from build123d import *

# Parameters (mm, degrees)
CYLINDER1964_R               = 1.5
CYLINDER1964_DEPTH           = 50
CYLINDER1964_PLACEMENT_ANGLE = 45
CYLINDER1965_R               = 1.5
CYLINDER1965_DEPTH           = 50
CYLINDER1965_PLACEMENT_ANGLE = 45
CYLINDER1963_R               = 1.5
CYLINDER1963_DEPTH           = 50
CYLINDER1963_PLACEMENT_ANGLE = 45
CYLINDER1962_R               = 1.5
CYLINDER1962_DEPTH           = 50
CYLINDER1962_PLACEMENT_ANGLE = 45
CYLINDER1967_R               = 1.5
CYLINDER1967_DEPTH           = 50
CYLINDER1967_PLACEMENT_ANGLE = 45
CYLINDER1966_R               = 1.5
CYLINDER1966_DEPTH           = 50
CYLINDER1966_PLACEMENT_ANGLE = 45
CYLINDER1954_R               = 3
CYLINDER1954_DEPTH           = 3
CYLINDER1954_PLACEMENT_ANGLE = 45
CYLINDER1953_R               = 3
CYLINDER1953_DEPTH           = 3
CYLINDER1953_PLACEMENT_ANGLE = 45
CYLINDER1955_R               = 3
CYLINDER1955_DEPTH           = 3
CYLINDER1955_PLACEMENT_ANGLE = 45
CYLINDER1952_R               = 3
CYLINDER1952_DEPTH           = 3
CYLINDER1952_PLACEMENT_ANGLE = 45
CYLINDER1950_R               = 3
CYLINDER1950_DEPTH           = 3
CYLINDER1950_PLACEMENT_ANGLE = 45
CYLINDER1951_R               = 3
CYLINDER1951_DEPTH           = 3
CYLINDER1951_PLACEMENT_ANGLE = 45
CYLINDER1936_R               = 8
CYLINDER1936_DEPTH           = 6
BOX803_W                     = 148
BOX803_H                     = 40
BOX803_DEPTH                 = 40
CYLINDER1935_R               = 34
CYLINDER1935_DEPTH           = 6
CHAMFER065_SIZE              = 2


with BuildPart() as obj1:
    # Cylinder1964 → Cylinder1964 (new body)
    with BuildSketch(Plane.XY):
        Circle(CYLINDER1964_R)
    extrude(amount=CYLINDER1964_DEPTH)


with BuildPart() as obj1_1:
    # Cylinder1964 placement: moved
    add(obj1.part.moved(Location((20, 137, 0))).rotate(Axis((20, 137, 0), (0, 0, 1)), CYLINDER1964_PLACEMENT_ANGLE))


with BuildPart() as compound991:
    # Cylinder1965 → Cylinder1965 (new body)
    with BuildSketch(Plane.XY):
        Circle(CYLINDER1965_R)
    extrude(amount=CYLINDER1965_DEPTH)


with BuildPart() as compound991_1:
    # Cylinder1965 placement: moved
    add(compound991.part.moved(Location((-20, 137, 0))).rotate(Axis((-20, 137, 0), (0, 0, 1)), CYLINDER1965_PLACEMENT_ANGLE))

    # Compound991: union obj1
    add(obj1_1.part)


with BuildPart() as obj2:
    # Cylinder1963 → Cylinder1963 (new body)
    with BuildSketch(Plane.XY):
        Circle(CYLINDER1963_R)
    extrude(amount=CYLINDER1963_DEPTH)


with BuildPart() as obj2_1:
    # Cylinder1963 placement: moved
    add(obj2.part.moved(Location((31, 131, 0))).rotate(Axis((31, 131, 0), (0, 0, 1)), CYLINDER1963_PLACEMENT_ANGLE))


with BuildPart() as compound992:
    # Cylinder1962 → Cylinder1962 (new body)
    with BuildSketch(Plane.XY):
        Circle(CYLINDER1962_R)
    extrude(amount=CYLINDER1962_DEPTH)


with BuildPart() as compound992_1:
    # Cylinder1962 placement: moved
    add(compound992.part.moved(Location((-31, 131, 0))).rotate(Axis((-31, 131, 0), (0, 0, 1)), CYLINDER1962_PLACEMENT_ANGLE))

    # Compound992: union obj2
    add(obj2_1.part)


with BuildPart() as obj3:
    # Cylinder1967 → Cylinder1967 (new body)
    with BuildSketch(Plane.XY):
        Circle(CYLINDER1967_R)
    extrude(amount=CYLINDER1967_DEPTH)


with BuildPart() as obj3_1:
    # Cylinder1967 placement: moved
    add(obj3.part.moved(Location((31, 101, 0))).rotate(Axis((31, 101, 0), (0, 0, 1)), CYLINDER1967_PLACEMENT_ANGLE))


with BuildPart() as compound994:
    # Cylinder1966 → Cylinder1966 (new body)
    with BuildSketch(Plane.XY):
        Circle(CYLINDER1966_R)
    extrude(amount=CYLINDER1966_DEPTH)


with BuildPart() as compound994_1:
    # Cylinder1966 placement: moved
    add(compound994.part.moved(Location((-31, 101, 0))).rotate(Axis((-31, 101, 0), (0, 0, 1)), CYLINDER1966_PLACEMENT_ANGLE))

    # Compound993: union obj3
    add(obj3_1.part)

    # Compound994: union Compound991, Compound992
    add(compound991_1.part)
    add(compound992_1.part)


with BuildPart() as obj4:
    # Cylinder1954 → Cylinder1954 (new body)
    with BuildSketch(Plane.XY):
        Circle(CYLINDER1954_R)
    extrude(amount=CYLINDER1954_DEPTH)


with BuildPart() as obj4_1:
    # Cylinder1954 placement: moved
    add(obj4.part.moved(Location((31, 131, 0))).rotate(Axis((31, 131, 0), (0, 0, 1)), CYLINDER1954_PLACEMENT_ANGLE))


with BuildPart() as compound982:
    # Cylinder1953 → Cylinder1953 (new body)
    with BuildSketch(Plane.XY):
        Circle(CYLINDER1953_R)
    extrude(amount=CYLINDER1953_DEPTH)


with BuildPart() as compound982_1:
    # Cylinder1953 placement: moved
    add(compound982.part.moved(Location((-31, 131, 0))).rotate(Axis((-31, 131, 0), (0, 0, 1)), CYLINDER1953_PLACEMENT_ANGLE))

    # Compound982: union obj4
    add(obj4_1.part)


with BuildPart() as compound982_2:
    # Compound982 placement: moved
    add(compound982_1.part.moved(Location((0, 0, 25))))


with BuildPart() as obj5:
    # Cylinder1955 → Cylinder1955 (new body)
    with BuildSketch(Plane.XY):
        Circle(CYLINDER1955_R)
    extrude(amount=CYLINDER1955_DEPTH)


with BuildPart() as obj5_1:
    # Cylinder1955 placement: moved
    add(obj5.part.moved(Location((31, 101, 0))).rotate(Axis((31, 101, 0), (0, 0, 1)), CYLINDER1955_PLACEMENT_ANGLE))


with BuildPart() as compound984:
    # Cylinder1952 → Cylinder1952 (new body)
    with BuildSketch(Plane.XY):
        Circle(CYLINDER1952_R)
    extrude(amount=CYLINDER1952_DEPTH)


with BuildPart() as compound984_1:
    # Cylinder1952 placement: moved
    add(compound984.part.moved(Location((-31, 101, 0))).rotate(Axis((-31, 101, 0), (0, 0, 1)), CYLINDER1952_PLACEMENT_ANGLE))

    # Compound984: union obj5
    add(obj5_1.part)


with BuildPart() as compound984_2:
    # Compound984 placement: moved
    add(compound984_1.part.moved(Location((0, 0, 21))))


with BuildPart() as obj6:
    # Cylinder1950 → Cylinder1950 (new body)
    with BuildSketch(Plane.XY):
        Circle(CYLINDER1950_R)
    extrude(amount=CYLINDER1950_DEPTH)


with BuildPart() as obj6_1:
    # Cylinder1950 placement: moved
    add(obj6.part.moved(Location((20, 137, 0))).rotate(Axis((20, 137, 0), (0, 0, 1)), CYLINDER1950_PLACEMENT_ANGLE))


with BuildPart() as compound985:
    # Cylinder1951 → Cylinder1951 (new body)
    with BuildSketch(Plane.XY):
        Circle(CYLINDER1951_R)
    extrude(amount=CYLINDER1951_DEPTH)


with BuildPart() as compound985_1:
    # Cylinder1951 placement: moved
    add(compound985.part.moved(Location((-20, 137, 0))).rotate(Axis((-20, 137, 0), (0, 0, 1)), CYLINDER1951_PLACEMENT_ANGLE))

    # Compound983: union obj6
    add(obj6_1.part)


with BuildPart() as compound985_2:
    # Compound983 placement: moved
    add(compound985_1.part.moved(Location((0, 0, 25))))

    # Compound985: union Compound982, Compound984
    add(compound982_2.part)
    add(compound984_2.part)


with BuildPart() as obj7:
    # Cylinder1936 → Cylinder1936 (new body)
    with BuildSketch(Plane(origin=(0, 83, 25), x_dir=(1, 0, 0), z_dir=(0, 0, 1))):
        Circle(CYLINDER1936_R)
    extrude(amount=CYLINDER1936_DEPTH)


with BuildPart() as krychle803:
    # Box803 → Box803 (new body)
    with BuildSketch(Plane(origin=(-74, 46, 16), x_dir=(1, 0, 0), z_dir=(0, 0, 1))):
        with Locations((74, 20)):
            Rectangle(BOX803_W, BOX803_H)
    extrude(amount=BOX803_DEPTH)


with BuildPart() as cut622:
    # Cylinder1935 → Cylinder1935 (new body)
    with BuildSketch(Plane(origin=(0, 101, 21), x_dir=(1, 0, 0), z_dir=(0, 0, 1))):
        Circle(CYLINDER1935_R)
    extrude(amount=CYLINDER1935_DEPTH)

    # Cut615: cut Krychle803
    add(krychle803.part, mode=Mode.SUBTRACT)

    # Cut616: cut obj7
    add(obj7.part, mode=Mode.SUBTRACT)

    # Chamfer065
    chamfer065_edges = [cut622.edges().sort_by_distance(p)[0] for p in [
        (-7.700067, 134.116597, 21),
    ]]
    chamfer(chamfer065_edges, length=CHAMFER065_SIZE)

    # Cut619: cut Compound985
    add(compound985_2.part, mode=Mode.SUBTRACT)

    # Cut622: cut Compound994
    add(compound994_1.part, mode=Mode.SUBTRACT)


solid = cut622.part
Verification items for the finished model (mm, model axes). A direction names the side the tool comes from. Round coordinates to 2 decimals unless told otherwise and drop trailing zeros. Write each loop counter-clockwise with the first axis right and the second up, starting at its lowest first coordinate (ties: lowest second). Pieces come first, ordered by that corner, then holes.
(1) Section check A-A (x = 0). Enter the section's corners in (y, z).
Returned:
outline: (86, 21) - (133, 21) - (135, 23) - (135, 27) - (91, 27) - (91, 25) - (86, 25) - close
(2) Access from +Z, -Z, +X, -X, +Y, -Y to the whole of each face (thin tool, end or side, straight path). Record for faces 1 (the flat face through (0, 86, 24)), 2 (the flat face through (0, 88, 25)), 3 (the flat face through (33, 101, 24)).
Returned:
face 1: +Z, -Z, +X, -X, -Y
face 2: +Z, -Y
face 3: -Z
(3) Material ranges on line 1 (X direction, y = 101, z = 24.65); line 2 (X direction, y = 98.5, z = 23.5); line 3 (Y direction, x = 1, z = 24.5), recorded low to high.
Returned:
line 1: x = -34 to -32.5, -29.5 to 29.5, 32.5 to 34
line 2: x = -33.91 to -32.66, -29.34 to 29.34, 32.66 to 33.91
line 3: y = 86 to 134.99
(4) Mould release check, pull along Y, two halves, no side actions. Record for faces 4 (the conical face through (31.767, 92.978, 21.764)), 5 (the cylindrical face through (0.965, 134.986, 24.972)), 6 (the cylindrical face through (-31.196, 99.513, 25.479)): pulls with the +Y half, pulls with the -Y half, needs draft (parallel to the pull), parting line crosses it, or undercut.
Returned:
face 4: pulls with the -Y half
face 5: parting line crosses it
face 6: undercut
(5) Depth check by flat-ended pin: pin 1 Ø4 at (x, y) = (25.5, 120.5) entering from -Z; pin 2 Ø5.5 at (x, y) = (-31, 101) entering from -Z; pin 3 Ø1 at (x, z) = (13, 22) entering from +Y; pin 4 Ø1.5 at (x, z) = (1, 23.5) entering from +Y. Enter the tip coordinate at first touch or a pass-through.
Returned:
pin 1: stops at z = 21
pin 2: stops at z = 24
pin 3: stops at y = 131.91
pin 4: stops at y = 135
